Geometry: final body of the model. Coordinates: model frame, mm. Coordinates: 2 decimals unless noted, no trailing zeros. Loops run counter-clockwise (first coordinate to the right, second up) from the corner with the lowest first, then second, coordinate; pieces in that order, holes last. Notation, with made-up numbers: (27.5, 73.5) -> (77.5, 73.5) arc R23 ccw to (77.5, 107.5) -> close; hole circle Ø8 at (-8, 49). An arc over 180 degrees is marked (long way). One line per item, written item: value. Start each with the question number.
from build123d import *

# Parameters (mm, degrees)
BOSS_EXTRUDE2_DEPTH = 3
SKETCH3_R           = 2.1
CUT_EXTRUDE3_DEPTH  = 4


with BuildPart() as part:
    # Sketch1 → Boss-Extrude2 (new body)
    with BuildSketch(Plane(origin=(0, 0, 0), x_dir=(1, 0, 0), z_dir=(0, 1, 0))):
        with BuildLine():
            Line((20, -5), (-20, -5))
            ThreePointArc((-20, -5), (-25, 0), (-20, 5))
            Line((-20, 5), (20, 5))
            ThreePointArc((20, 5), (25, 0), (20, -5))
        make_face()
    extrude(amount=BOSS_EXTRUDE2_DEPTH)

    # Sketch3 → Cut-Extrude3 (cut, through all)
    with BuildSketch(Plane(origin=(0, 3, 0), x_dir=(1, 0, 0), z_dir=(0, 1, 0))):
        with Locations(Location((-20, 0, 0), (0, 0, 270))):  # turned: the seam where the file's is
            Circle(SKETCH3_R)
    cut_extrude3 = extrude(amount=-CUT_EXTRUDE3_DEPTH, mode=Mode.SUBTRACT)

    # Mirror1: Cut-Extrude3 across plane
    add(cut_extrude3.mirror(Plane(origin=(0, 0, 0), x_dir=(0, 0, 1), z_dir=(1, 0, 0))), mode=Mode.SUBTRACT)


solid = part.part
1. Draft query along Z for faces 1 (the face through (-18.23, 1.52, 1.13)), 2 (the face through (0, 1, -5)), 3 (the face through (-25, 1, 0)). Return one class per face: released by +Z, released by -Z, zero draft, split by the parting line, or undercut.
2. Section C-C on z = 4.25. Return the cut outline in (x, y), plus the area to 3 significant figures.
3. Section A-A on z = 0. Return the cut outline in (x, y).
4. Line query: L1, parallel to X at y = 1.6, z = 0; L2, parallel to X at y = 1.75, z = -0.5; L3, parallel to Z at x = -19, y = 0.6. Output: solid intervals per line, ascending. Write a range as [from, to].
5. Section B-B on y = 1.1. Return the cut outline in (x, z).
6. Pin query (flat end, axial travel): pin 1 Ø3.5 at (x, z) = (-20, 0) entering from -Y. Return the tip coordinate at first contact, or that it passes through.
Checks:
1. face 1: undercut
1. face 2: released by -Z
1. face 3: split by the parting line
2. outline: (-22.63, 0) -> (22.63, 0) -> (22.63, 3) -> (-22.63, 3) -> close
2. area: 136 mm²
3. outline: (-25, 0) -> (-22.1, 0) -> (-22.1, 3) -> (-25, 3) -> close; (-17.9, 0) -> (17.9, 0) -> (17.9, 3) -> (-17.9, 3) -> close; (22.1, 0) -> (25, 0) -> (25, 3) -> (22.1, 3) -> close
4. L1: [-25, -22.1], [-17.9, 17.9], [22.1, 25]
4. L2: [-24.97, -22.04], [-17.96, 17.96], [22.04, 24.97]
4. L3: [-5, -1.85], [1.85, 5]
5. outline: (-20, -5) -> (20, -5) arc R5 ccw to (20, 5) -> (-20, 5) arc R5 ccw to start; hole circle Ø4.2 at (-20, 0); hole circle Ø4.2 at (20, 0)
6. pin 1: through
